Could you check a few things on this model? Use its own coordinates, in mm. A direction names the side the tool comes from. Coordinates: 2 decimals unless noted, no trailing zeros. Order: outer loops, then holes, each group sorted by start corner. A loop starts at its lowest first (then second) coordinate and runs counter-clockwise, first axis right, second up. Notation, with made-up numbers: (39, 47.25) - (82, 47.25) arc R11 cw to (82, 56.25) - close; hole circle Ø8 at (56, 80). An arc over 180 degrees is marked (long way). One line per item, written item: value.
Autodesk Inventor part; units mm, degrees
ref_plane "YZ Plane" through (0, 0, 0) normal (1, 0, 0) x (0, 1, 0)
ref_plane "XZ Plane" through (0, 0, 0) normal (0, 1, 0) x (-1, 0, 0)
ref_plane "XY Plane" through (0, 0, 0) normal (0, 0, 1) x (1, 0, 0)
sketch "Sketch1" plane through (0, 0, 0) normal (0, 0, 1) x (1, 0, 0)
  line L0 (3.175, 0) -> (146.685, 0)
  line L1 (149.86, 161.925) -> (0, 161.925)
  line L2 (0, 161.925) -> (3.175, 0)
  line L3 (149.86, 161.925) -> (146.685, 0)
  point P0 (0, 0)
  dimension "d74" = 161.925
  dimension "d75" = 143.51
  dimension "d76" = 149.86
extrude "Extrusion1" add sketch "Sketch1" along normal blind 3.048
fillet "Fillet1" radius 6.35 3 edges at (149.86, 161.925, 1.524) (146.685, 0, 1.524) (0, 161.925, 1.524)
fillet "Fillet4" radius 6.35 1 edges at (3.175, 0, 1.524)
sketch "Sketch21" plane through (0, 0, 3.048) normal (0, 0, 1) x (1, 0, 0)
  arc A0 (149.733, 155.4505) -> (143.3843, 161.925) centre (143.3843, 155.575) ccw
  line L0 (143.3843, 139.7) -> (143.3843, 152.4)
  line L1 (6.4757, 152.4) -> (6.4757, 139.7)
  line L2 (79.8843, 152.4) -> (79.8843, 139.7)
  line L3 (69.9757, 152.4) -> (69.9757, 139.7)
  line L4 (140.2093, 155.575) -> (83.0593, 155.575)
  line L5 (66.8007, 155.575) -> (9.6507, 155.575)
  line L6 (9.6507, 136.525) -> (66.8007, 136.525)
  line L7 (83.0593, 136.525) -> (140.2093, 136.525)
  arc A1 (9.6507, 155.575) -> (6.4757, 152.4) centre (9.6507, 152.4) ccw
  arc A2 (6.4757, 139.7) -> (9.6507, 136.525) centre (9.6507, 139.7) ccw
  arc A3 (66.8007, 136.525) -> (69.9757, 139.7) centre (66.8007, 139.7) ccw
  arc A4 (69.9757, 152.4) -> (66.8007, 155.575) centre (66.8007, 152.4) ccw
  arc A5 (83.0593, 155.575) -> (79.8843, 152.4) centre (83.0593, 152.4) ccw
  arc A6 (79.8843, 139.7) -> (83.0593, 136.525) centre (83.0593, 139.7) ccw
  arc A7 (140.2093, 136.525) -> (143.3843, 139.7) centre (140.2093, 139.7) ccw
  arc A8 (143.3843, 152.4) -> (140.2093, 155.575) centre (140.2093, 152.4) ccw
  line L8 (137.6362, 22.225) -> (137.6362, 9.525)
  line L9 (12.2237, 9.525) -> (12.2237, 22.225)
  line L10 (12.2237, 25.4) -> (137.6362, 6.35) construction
  line L11 (137.6362, 25.4) -> (12.2237, 6.35) construction
  line L12 (69.9757, 9.525) -> (69.9757, 22.225)
  line L13 (79.8843, 22.225) -> (79.8843, 9.525)
  line L14 (79.8843, 6.35) -> (69.9757, 25.4) construction
  line L15 (69.9757, 6.35) -> (79.8843, 25.4) construction
  line L16 (15.3987, 25.4) -> (66.8007, 25.4)
  line L17 (83.0593, 25.4) -> (134.4612, 25.4)
  line L18 (134.4612, 6.35) -> (83.0593, 6.35)
  line L19 (66.8007, 6.35) -> (15.3987, 6.35)
  arc A9 (15.3987, 25.4) -> (12.2237, 22.225) centre (15.3987, 22.225) ccw
  arc A10 (12.2237, 9.525) -> (15.3987, 6.35) centre (15.3987, 9.525) ccw
  arc A11 (66.8007, 6.35) -> (69.9757, 9.525) centre (66.8007, 9.525) ccw
  arc A12 (69.9757, 22.225) -> (66.8007, 25.4) centre (66.8007, 22.225) ccw
  arc A13 (83.0593, 25.4) -> (79.8843, 22.225) centre (83.0593, 22.225) ccw
  arc A14 (137.6362, 22.225) -> (134.4612, 25.4) centre (134.4612, 22.225) ccw
  arc A15 (134.4612, 6.35) -> (137.6362, 9.525) centre (134.4612, 9.525) ccw
  arc A16 (79.8843, 9.525) -> (83.0593, 6.35) centre (83.0593, 9.525) ccw
  point P0 (0, 0)
  point P1 (74.93, 15.875)
  dimension "d97" = 3.175
  dimension "d111" = 19.05
  dimension "d112" = 19.05
  dimension "d113" = 63.5
  dimension "d114" = 63.5
  dimension "d131" = 9.9085
  dimension "d141" = 19.05
  dimension "d142" = 3.175
extrude "Extrusion20" cut sketch "Sketch21" against normal blind 3.048
sketch "Sketch23" plane through (0, 0, 3.048) normal (0, 0, 1) x (1, 0, 0)
  line L0 (142.875, 27.752) -> (6.985, 27.752)
  line L1 (6.985, 27.752) -> (6.985, 133.924)
  line L2 (6.985, 133.924) -> (142.875, 133.924)
  line L3 (142.875, 133.924) -> (142.875, 27.752)
  line L4 (142.875, 27.752) -> (6.985, 133.924) construction
  line L5 (6.985, 27.752) -> (142.875, 133.924) construction
  line L6 (10.16, 130.749) -> (139.7, 130.749)
  line L7 (10.16, 30.927) -> (10.16, 130.749)
  line L8 (139.7, 30.927) -> (10.16, 30.927)
  line L9 (139.7, 130.749) -> (139.7, 30.927)
  point P0 (0, 0)
  point P1 (74.93, 80.838)
  dimension "d129" = 135.89
  dimension "d130" = 106.172
  dimension "d132" = 3.175
  dimension "d133" = 3.175
  dimension "d134" = 3.175
  dimension "d135" = 3.175
extrude "Extrusion22" cut sketch "Sketch23" against normal blind 3.048 contours L6 L9 L8 L7
sketch "Sketch25" plane through (0, 0, 3.048) normal (0, 0, 1) x (1, 0, 0)
  line L0 (10.16, 30.927) -> (10.16, 130.749)
  line L1 (10.16, 130.749) -> (139.7, 130.749)
  line L2 (139.7, 130.749) -> (139.7, 30.927)
  line L3 (139.7, 30.927) -> (10.16, 30.927)
  line L4 (142.875, 133.924) -> (6.985, 133.924)
  line L5 (6.985, 133.924) -> (6.985, 27.752)
  line L6 (6.985, 27.752) -> (142.875, 27.752)
  line L7 (142.875, 27.752) -> (142.875, 133.924)
  point P0 (0, 0)
  dimension "d138" = 3.175
extrude "Extrusion23" cut sketch "Sketch25" against normal blind 1.27
sketch "Sketch34" plane through (0, 0, 0) normal (0, 0, -1) x (-1, 0, 0)
  line L0 (-10.16, 130.749) -> (-10.16, 30.927)
  line L1 (-10.16, 30.927) -> (-139.7, 30.927)
  line L2 (-139.7, 30.927) -> (-139.7, 130.749)
  line L3 (-139.7, 130.749) -> (-10.16, 130.749)
  line L4 (-6.985, 133.924) -> (-6.985, 27.752)
  line L5 (-6.985, 27.752) -> (-142.875, 27.752)
  line L6 (-142.875, 27.752) -> (-142.875, 133.924)
  line L7 (-142.875, 133.924) -> (-6.985, 133.924)
  circle A0 centre (-134.9375, 113.35) radius 2.413
  line L8 (-129.3495, 117.923) -> (-129.3495, 108.777)
  line L9 (-130.8642, 120.6293) -> (-138.1853, 125.1208)
  line L10 (-130.8642, 106.0708) -> (-138.1853, 101.5793)
  line L11 (-139.7, 127.827) -> (-139.7, 130.749)
  line L12 (-139.7, 98.873) -> (-139.7, 93.6625)
  arc A1 (-139.7, 127.827) -> (-138.1853, 125.1208) centre (-136.525, 127.827) ccw
  arc A2 (-129.3495, 117.923) -> (-130.8642, 120.6293) centre (-132.5245, 117.923) ccw
  arc A3 (-130.8642, 106.0708) -> (-129.3495, 108.777) centre (-132.5245, 108.777) ccw
  arc A4 (-138.1853, 101.5793) -> (-139.7, 98.873) centre (-136.525, 98.873) ccw
  line L13 (-139.7, 127.827) -> (-139.7, 98.873)
  circle A5 centre (-25.654, 35.6895) radius 2.413
  line L14 (-21.081, 41.275) -> (-30.227, 41.275)
  line L15 (-32.9333, 39.7603) -> (-37.4232, 32.4417)
  line L16 (-18.3747, 39.7603) -> (-13.8848, 32.4417)
  line L17 (-40.1295, 30.927) -> (-42.8625, 30.927)
  line L18 (-11.1785, 30.927) -> (-10.16, 30.927)
  arc A6 (-40.1295, 30.927) -> (-37.4232, 32.4417) centre (-40.1295, 34.102) ccw
  arc A7 (-13.8848, 32.4417) -> (-11.1785, 30.927) centre (-11.1785, 34.102) ccw
  arc A8 (-18.3747, 39.7603) -> (-21.081, 41.275) centre (-21.081, 38.1) ccw
  arc A9 (-30.227, 41.275) -> (-32.9333, 39.7603) centre (-30.227, 38.1) ccw
  line L19 (-40.1295, 30.927) -> (-11.1785, 30.927)
  point P0 (0, 0)
  point P1 (-129.3495, 119.7)
  point P2 (-129.3495, 107)
  point P3 (-139.7, 126.05)
  point P4 (-139.7, 100.65)
  point P5 (-19.304, 41.275)
  point P6 (-32.004, 41.275)
  point P7 (-38.3525, 30.927)
  point P8 (-12.9555, 30.927)
  dimension "d223" = 3.175
  dimension "d226" = 4.826
  dimension "d227" = 20.574
  dimension "d228" = 7.9375
  dimension "d231" = 12.7
  dimension "d235" = 3.175
  dimension "d240" = 4.826
  dimension "d241" = 18.669
  dimension "d242" = 7.9375
  dimension "d244" = 12.7
  dimension "d247" = 3.175
  dimension "d248" = 8.127
  dimension "d249" = 8.127
  dimension "d250" = 4.573
  dimension "d251" = 4.573
  dimension "d253" = 5.588
  dimension "d254" = 4.573
  dimension "d255" = 4.573
extrude "Extrusion29" add sketch "Sketch34" against normal blind 1.778 contours L1 A6 L15 A9 L14 A8 L16 A7 | A1 L9 A2 L8 A3 L10 A4 L2
properties part number "control pod layer b"
Item 1: I want a section at C-C on y = 53. Please give me the cut outline in (x, z) (3 decimals).
Conclusion:
outline: (2.136, 0) - (10.16, 0) - (10.16, 1.778) - (6.985, 1.778) - (6.985, 3.048) - (2.136, 3.048) - close; (139.7, 0) - (147.724, 0) - (147.724, 3.048) - (142.875, 3.048) - (142.875, 1.778) - (139.7, 1.778) - close
Item 2: If I drill on probe 1 along Y at (x, z) = (60, 2.9) (3 decimals); probe 2 along Y at (x, z) = (128.5, 0.95) (3 decimals); probe 3 along Y at (x, z) = (140.5, 1.4) (3 decimals), over which ranges is the centre line in solid material (lowest first)?
Conclusion:
probe 1: 0 to 6.35, 25.4 to 27.752, 133.924 to 136.525, 155.575 to 161.925
probe 2: 0 to 6.35, 25.4 to 30.927, 130.749 to 136.525, 155.575 to 161.925
probe 3: 0 to 136.538, 155.562 to 161.925
Item 3: I'm going to push flat-ended pins straight in: pin 1 Ø1.4 at (y, z) = (128.5, 0.5) entering from -X; pin 2 Ø1.5 at (y, z) = (14, 1.5) entering from +X; pin 3 Ø0.9 at (y, z) = (19, 1.5) entering from -X. Where does each tip first touch, or does it pass through?
Conclusion:
pin 1: x = 0.64
pin 2: x = 146.97
pin 3: x = 2.79
Item 4: I want a section at A-A on x = 72.5. Please give me the cut outline in (y, z) (3 decimals), then the cut area to 3 significant figures.
Conclusion:
outline: (0, 0) - (30.927, 0) - (30.927, 1.778) - (27.752, 1.778) - (27.752, 3.048) - (0, 3.048) - close; (130.749, 0) - (161.925, 0) - (161.925, 3.048) - (133.924, 3.048) - (133.924, 1.778) - (130.749, 1.778) - close
area: 181 mm²
Item 5: For faces 4 (the face through (16.16, 36.15, 0.88)), 5 (the face through (4.91, 1.86, 1.55)), which set-ups out of +Z, -Z, +X, -X, +Y, -Y let a thin tool reach every point of the face, with its end or its side?
Conclusion:
face 4: +Z, -Z
face 5: +Z, -Z, -X, -Y
Item 6: I want a section at D-D on y = 113.35. Please give me the cut outline in (x, z) (1 decimal), then the cut area to 3 significant figures.
Conclusion:
outline: (1, 0) - (10.2, 0) - (10.2, 1.8) - (7, 1.8) - (7, 3) - (1, 3) - close; (129.3, 0) - (132.5, 0) - (132.5, 1.8) - (129.3, 1.8) - close; (137.4, 0) - (148.9, 0) - (148.9, 3) - (142.9, 3) - (142.9, 1.8) - (137.4, 1.8) - close
area: 57.9 mm²
Item 7: I want a section at B-B on x = 89.5. Please give me the cut outline in (y, z) (3 decimals), then the cut area to 3 significant figures.
Conclusion:
outline: (0, 0) - (6.35, 0) - (6.35, 3.048) - (0, 3.048) - close; (25.4, 0) - (30.927, 0) - (30.927, 1.778) - (27.752, 1.778) - (27.752, 3.048) - (25.4, 3.048) - close; (130.749, 0) - (136.525, 0) - (136.525, 3.048) - (133.924, 3.048) - (133.924, 1.778) - (130.749, 1.778) - close; (155.575, 0) - (161.925, 0) - (161.925, 3.048) - (155.575, 3.048) - close
area: 65.1 mm²
Item 8: Thinking about a two-plate mould opening in X: for faces 1 (the face through (63, 27, 3.048)), 2 (the face through (75, 132, 1.778)), 3 (the face through (144.855, 1.768, 1.545)), which applies, pulls with the +X half, pulls with the -X half, needs draft (parallel to the pull), parting line crosses it, or undercut?
Conclusion:
face 1: needs draft
face 2: undercut
face 3: pulls with the +X half
